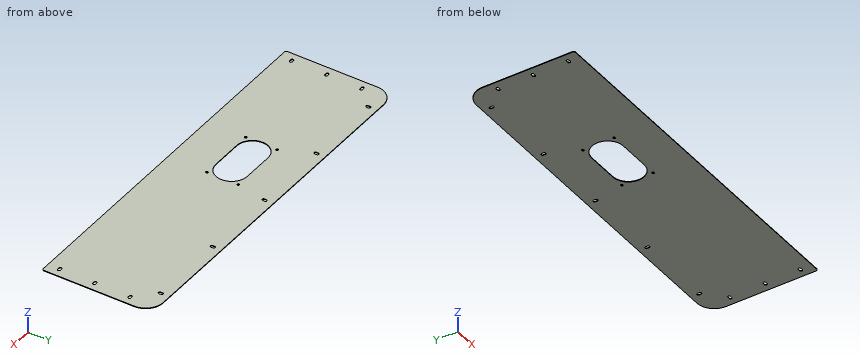
from build123d import *

# Parameters (mm, degrees)
SKETCH_1_W             = 939
SKETCH_1_H             = 280
SM_BASE_FLANGE_1_DEPTH = 1.5
CUT_EXTRUDE_1_DEPTH    = 10
FILLET_1_R             = 45
FILLET_2_R             = 5
CUT_EXTRUDE_2_DEPTH    = 10
PATTERN_LINEAR_1_COUNT = 5
PATTERN_LINEAR_1_PITCH = 200
CUT_EXTRUDE_3_DEPTH    = 10
PATTERN_LINEAR_2_COUNT = 3
PATTERN_LINEAR_2_PITCH = 90
SKETCH_36_R            = 3
CUT_EXTRUDE_4_DEPTH    = 10


# Sheet-metal steps are written as plain solids
with BuildPart() as part:
    # Sketch 1 → 基体-法兰1 (new body)
    with BuildSketch(Plane.XY):
        Rectangle(SKETCH_1_W, SKETCH_1_H)
    extrude(amount=-SM_BASE_FLANGE_1_DEPTH)

    # 草图33 → 切除-拉伸1 (cut)
    with BuildSketch(Plane(origin=(0, 0, -1.5), x_dir=(-1, 0, 0), z_dir=(0, 0, -1))):
        with BuildLine():
            Line((50, 40), (130, 40))
            ThreePointArc((130, 40), (170, 0), (130, -40))
            Line((130, -40), (50, -40))
            ThreePointArc((50, -40), (10, 0), (50, 40))
        make_face()
    extrude(amount=-CUT_EXTRUDE_1_DEPTH, mode=Mode.SUBTRACT)

    # 圆角1
    fillet_1_edges = [part.edges().sort_by_distance(p)[0] for p in [
        (-469.5, 140, -0.75),
        (469.5, 140, -0.75),
    ]]
    fillet(fillet_1_edges, radius=FILLET_1_R)

    # 圆角2
    fillet_2_edges = [part.edges().sort_by_distance(p)[0] for p in [
        (469.5, -140, -0.75),
        (-469.5, -140, -0.75),
    ]]
    fillet(fillet_2_edges, radius=FILLET_2_R)

    # 草图34 → 切除-拉伸2 (cut)
    with BuildSketch(Plane(origin=(0, 0, -1.5), x_dir=(-1, 0, 0), z_dir=(0, 0, -1))):
        with BuildLine():
            Line((-396.5, 120), (-396.5, 115))
            ThreePointArc((-396.5, 115), (-400, 111.5), (-403.5, 115))
            Line((-403.5, 115), (-403.5, 120))
            ThreePointArc((-403.5, 120), (-400, 123.5), (-396.5, 120))
        make_face()
    cut_extrude_2 = extrude(amount=-CUT_EXTRUDE_2_DEPTH, mode=Mode.SUBTRACT)

    # 阵列(线性)1: 切除-拉伸2 ×5
    with Locations(*[(-i * PATTERN_LINEAR_1_PITCH, 0, 0) for i in range(1, PATTERN_LINEAR_1_COUNT)]):
        add(cut_extrude_2, mode=Mode.SUBTRACT)

    # 草图35 → 切除-拉伸3 (cut)
    with BuildSketch(Plane(origin=(0, 0, -1.5), x_dir=(-1, 0, 0), z_dir=(0, 0, -1))):
        with BuildLine():
            Line((-449.5, -106.5), (-444.5, -106.5))
            ThreePointArc((-444.5, -106.5), (-441, -110), (-444.5, -113.5))
            Line((-444.5, -113.5), (-449.5, -113.5))
            ThreePointArc((-449.5, -113.5), (-453, -110), (-449.5, -106.5))
        make_face()
        with BuildLine():
            Line((444.5, -106.5), (449.5, -106.5))
            ThreePointArc((449.5, -106.5), (453, -110), (449.5, -113.5))
            Line((449.5, -113.5), (444.5, -113.5))
            ThreePointArc((444.5, -113.5), (441, -110), (444.5, -106.5))
        make_face()
    cut_extrude_3 = extrude(amount=-CUT_EXTRUDE_3_DEPTH, mode=Mode.SUBTRACT)

    # 阵列(线性)2: 切除-拉伸3 ×3
    with Locations(*[(0, i * PATTERN_LINEAR_2_PITCH, 0) for i in range(1, PATTERN_LINEAR_2_COUNT)]):
        add(cut_extrude_3, mode=Mode.SUBTRACT)

    # 草图36 → 切除-拉伸4 (cut)
    with BuildSketch(Plane(origin=(0, 0, -1.5), x_dir=(-1, 0, 0), z_dir=(0, 0, -1))):
        with Locations((15, 40)):
            Circle(SKETCH_36_R)
        with Locations((165, 40)):
            Circle(SKETCH_36_R)
        with Locations((165, -40)):
            Circle(SKETCH_36_R)
        with Locations((15, -40)):
            Circle(SKETCH_36_R)
    extrude(amount=-CUT_EXTRUDE_4_DEPTH, mode=Mode.SUBTRACT)


solid = part.part
The model under review builds one solid part; all positions refer to its coordinate system, in mm. Coordinates: 2 decimals unless noted, no trailing zeros. Write each loop counter-clockwise with the first axis right and the second up, starting at its lowest first coordinate (ties: lowest second). Pieces come first, ordered by that corner, then holes. Notation, with made-up numbers: (6, -26) -> (12, -26) arc R16 ccw to (12, -5) -> close; hole circle Ø8 at (-8, -38). An arc over 180 degrees is marked (long way). Answer in a Markdown table with one row per item.
1. We need section A-A, the plane x = -27. State the section outline as (y, z) points.
Answers below:
| item | result |
|---|---|
| outline | (-140, -1.5) -> (-32.73, -1.5) -> (-32.73, 0) -> (-140, 0) -> close; (32.73, -1.5) -> (140, -1.5) -> (140, 0) -> (32.73, 0) -> close |
2. We need section B-B, the plane z = -0.9. Give the number of separate pieces and of enclosed holes in the cut face, and give its area (3 significant figures).
Answers below:
| item | result |
|---|---|
| separate pieces | 1 |
| enclosed holes | 16 |
| area | 250,000 mm^2 |
3. Clearance check with flat-ended pins moving along their axes: pin 1 Ø0.8 at (x, z) = (-447, -0.5) entering from +Y; pin 2 Ø0.8 at (y, z) = (117, -0.5) entering from -X; pin 3 Ø5 at (x, y) = (-15, 40) entering from -Z. State where each tip first meets the part, or that it passes through.
Answers below:
| item | result |
|---|---|
| pin 1 | stops at y = 134.2 |
| pin 2 | stops at x = -463.98 |
| pin 3 | passes through |
4. Wall thickness on probe 1 along X at (y, z) = (69, -1.25); probe 2 along Y at (x, z) = (-165, -1.15); probe 3 along X at (y, z) = (11, -1): over which ranges is each line inside the solid? List them lowest first. Write a range as [from, to].
Answers below:
| item | result |
|---|---|
| probe 1 | x = [-469.5, -452.85], [-441.15, 441.15], [452.85, 469.5] |
| probe 2 | y = [-140, -43], [-37, -19.36], [19.36, 37], [43, 140] |
| probe 3 | x = [-469.5, -168.46], [-11.54, 469.5] |
